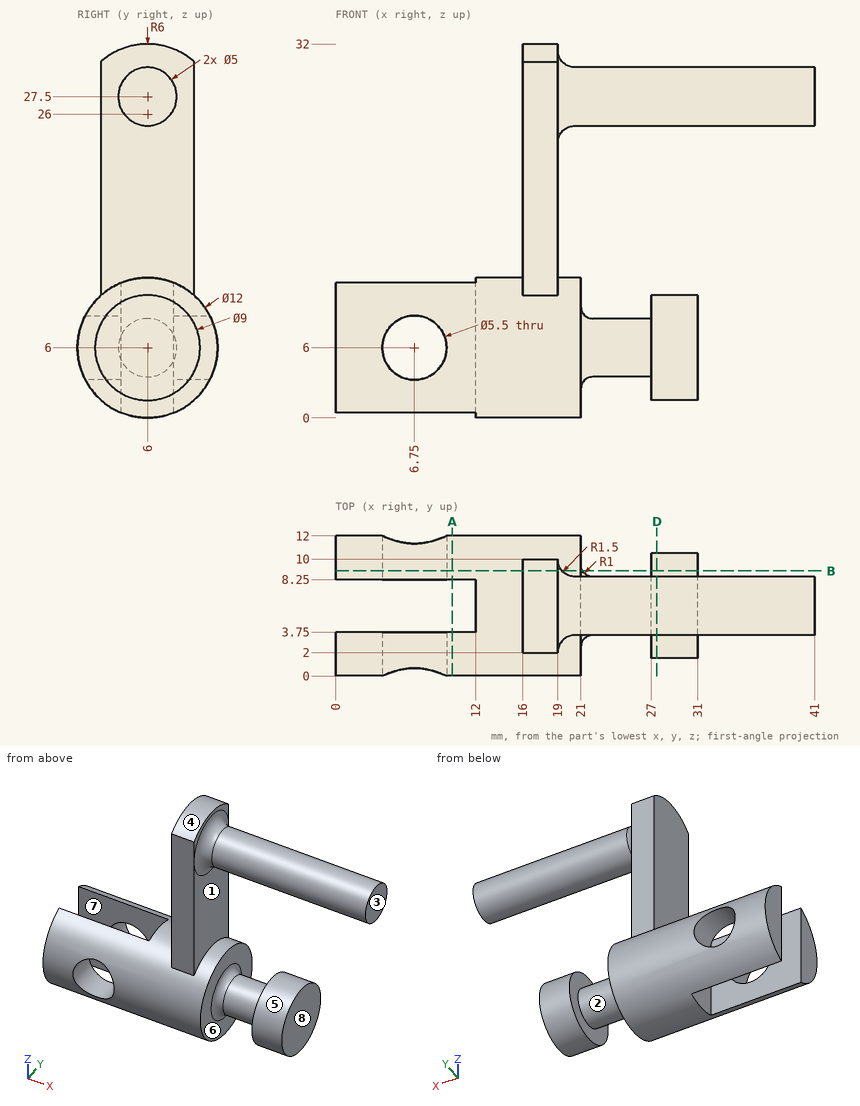
Job drawing, mm, ordinate dimensions from the low corner. One solid piece. A direction names the side the tool comes from. Coordinates: 2 decimals unless noted, no trailing zeros. Order: outer loops, then holes, each group sorted by start corner. A loop starts at its lowest first (then second) coordinate and runs counter-clockwise, first axis right, second up. Notation, with made-up numbers: (76.5, 75) -> (108.5, 75) arc R25 cw to (108.5, 101) -> close; hole circle Ø11 at (12.25, -13). An arc over 180 degrees is marked (long way). Put each result on its own line as item: value. Start each with the question number.
(1) Mould opens along Z. For the marked faces 1, 2, 3 and 4 say: pulls with the +Z half, pulls with the -Z half, needs draft (parallel to the pull), parting line crosses it, or undercut.
(2) Probe line 1 along X through (y, z) = (10, 6); line 2 along X through (y, z) = (1.2, 6); line 3 along X through (y, z) = (5.25, 22.5). List the from-to ranges inside material, lowest first. Write a range as [from, to].
(3) Band-saw the part on D-D (x = 27.5). Give the cut face in (y, z).
(4) Pin check, flat tips, straight feed: pin 1 Ø8 at (x, z) = (5, 11.5) entering from +Y; pin 2 Ø5 at (x, z) = (6.75, 6) entering from +Y; pin 3 Ø6 at (x, y) = (25.5, 2.5) entering from -Z; pin 4 Ø3.5 at (x, z) = (17.5, 25.5) entering from -Y. Stop position of each tip, or through.
(5) Which spindle directions (+Z, -Z, +X, -X, +Y, -Y) get a long thin tool onto all of the face, cutting with end or side? Do the marked faces 5, 6, 7 and 8. Say none if no direction does.
(6) Band-saw the part on B-B (y = 9). Count the separate pieces of the cut face and the enclosed holes in it, then the cut area to 3 significant figures.
(7) Band-saw the part on A-A (x = 10). Give the cut face in (y, z).
Determined:
1. face 1: undercut
1. face 2: undercut
1. face 3: needs draft
1. face 4: pulls with the +Z half
2. line 1: x = [0, 4], [9.5, 21], [27, 31]
2. line 2: x = [0, 4], [9.5, 21]
2. line 3: x = [16, 19]
3. outline: circle Ø9 at (6, 6); circle Ø5 at (6, 27.5)
4. pin 1: stops at y = 11.8
4. pin 2: passes through
4. pin 3: stops at z = 1.59
4. pin 4: stops at y = 2
5. face 5: +X
5. face 6: none
5. face 7: +Z, -Z, -X
5. face 8: -Z, +X, +Y, -Y
6. separate pieces: 2
6. enclosed holes: 1
6. area: 283 mm²
7. outline: (3.75, 0.44) -> (3.75, 11.56) arc R6 ccw to start; (8.25, 0.44) arc R6 ccw to (8.25, 11.56) -> close
